from build123d import *

# Parameters (mm, degrees)
F0_R     = 37.5
F1_DEPTH = 80
F2_T     = -4
F3_R     = 37.5
F3_R_2   = 35.5
F4_DEPTH = 15
F5_R     = 3


with BuildPart() as f1:
    # F0 (on Top) → F1 (new body)
    with BuildSketch(Plane.XY):
        Circle(F0_R)
    extrude(amount=F1_DEPTH)

    # F2
    f2_openings = [f1.faces().sort_by_distance(p)[0] for p in [
        (0, 0, 80),
    ]]
    offset(amount=F2_T, openings=f2_openings)

    # F3 (on face) → F4 (cut)
    with BuildSketch(Plane.XY.offset(80)):
        Circle(F3_R)
        Circle(F3_R_2, mode=Mode.SUBTRACT)
    extrude(amount=-F4_DEPTH, mode=Mode.SUBTRACT)

    # F5
    f5_edges = [f1.edges().sort_by_distance(p)[0] for p in [
        (-37.5, 0, 0),
        (-33.5, 0, 4),
    ]]
    fillet(f5_edges, radius=F5_R)


solid = f1.part
Verification items for the finished model (mm, model axes). A direction names the side the tool comes from. Coordinates: 2 decimals unless noted, no trailing zeros. Loops run counter-clockwise (first coordinate to the right, second up) from the corner with the lowest first, then second, coordinate; pieces in that order, holes last. Notation, with made-up numbers: (71, 59) -> (122, 59) arc R26 ccw to (122, 74) -> close; hole circle Ø6 at (-25.5, -12). An arc over 180 degrees is marked (long way). Answer as CSV lines item,"result".
1) Cross-section at C-C, the plane z = 71.5. Record the cut outline in (x, y).
Found:
outline,"circle Ø71 at (0, 0); hole circle Ø67 at (0, 0)"
2) Thickness scan on L1, parallel to Y at x = 0, z = 56.5; L2, parallel to Z at x = -9, y = -14; L3, parallel to Z at x = 21, y = 27.5. Record the ranges inside material, lowest first. Write a range as from..to.
Found:
L1,"y = -37.5..-33.5, 33.5..37.5"
L2,"z = 0..4"
L3,"z = 0..80"
3) Cross-section at D-D, the plane z = 25.5. Record the cut outline in (x, y), then the cut area to 3 significant figures.
Found:
outline,"circle Ø75 at (0, 0); hole circle Ø67 at (0, 0)"
area,"892 mm2"
4) Depth check by flat-ended pin: pin 1 (10 mm diameter, centred on y = -17.5, z = 40, fed in from +X); pin 2 (12 mm diameter, centred on x = -26, z = 49.5, fed in from -Y); pin 3 (2 mm diameter, centred on x = 20, y = 9.5, fed in from +Z). Enter the tip coordinate at first touch or a pass-through.
Found:
pin 1,"stops at x = 35.36"
pin 2,"stops at y = -31.72"
pin 3,"stops at z = 4"
5) Tool access check on faces 5 (the flat face through (33, -14, 65)), 6 (the flat face through (26.131, 21.203, 80)). Record the directions out of +Z, -Z, +X, -X, +Y, -Y that give a thin tool (end or side, any length) a straight path to the whole face; none if there is none.
Found:
face 5,"+Z"
face 6,"+Z, +X, -X, +Y, -Y"
6) Release check for a two-part mould opening along X. For faces 1 (the flat face through (0, 0, 4)), 2 (the flat face through (0, 0, 0)), 3 (the cylindrical face through (-7.262, -32.703, 42.989)), 4 (the cylindrical face through (-7.696, -34.656, 72.605)) record: +X half, -X half, draft (parallel to the pull), parting line (faces both ways), or undercut.
Found:
face 1,"undercut"
face 2,"draft"
face 3,"undercut"
face 4,"parting line"
7) Cross-section at A-A, the plane y = 0. Record the cut outline in (x, z), then the cut area to 3 significant figures.
Found:
outline,"(-37.5, 3) arc R3 ccw to (-34.5, 0) -> (34.5, 0) arc R3 ccw to (37.5, 3) -> (37.5, 65) -> (35.5, 65) -> (35.5, 80) -> (33.5, 80) -> (33.5, 7) arc R3 cw to (30.5, 4) -> (-30.5, 4) arc R3 cw to (-33.5, 7) -> (-33.5, 80) -> (-35.5, 80) -> (-35.5, 65) -> (-37.5, 65) -> close"
area,"848 mm2"
